Verification items for the finished model (mm, model axes). A direction names the side the tool comes from. Give positions to 0.01 mm unless a question says otherwise; leave off trailing zeros.
from build123d import *

# Parameters (mm, degrees)
SWEEP_1_PROFILE_R   = 10
SWEEP_1_PROFILE_R_2 = 7.5


with BuildPart() as part:
    # 扫描-薄件1: sweep along a curve in space
    with BuildLine() as sweep_1_path:
        Line((0, 0, 0), (0, 13.370069625, 0))
        ThreePointArc((0, 13.370069625, 0), (-3.799479767, 27.216391611, -1.753606046), (-13.925963802, 36.427367909, -6.427367909))
        Line((-51.074036198, 53.572632091, -23.572632091), (-13.925963802, 36.427367909, -6.427367909))
        ThreePointArc((-65, 60, -46.629930375), (-61.200520233, 58.246393954, -32.783608389), (-51.074036198, 53.572632091, -23.572632091))
        Line((-65, 60, -46.629930375), (-65, 60, -50))
    # 扫描-薄件1 profile (on start of the path) → 扫描-薄件1 (sweep)
    with BuildSketch(Plane(origin=(0, 0, 0), x_dir=(1, 0, 0), z_dir=(0, 1, 0))):
        Circle(SWEEP_1_PROFILE_R)
        Circle(SWEEP_1_PROFILE_R_2, mode=Mode.SUBTRACT)
    sweep(path=sweep_1_path.line)


solid = part.part
(1) Set-up check for faces 4 (the cylindrical face through (-7.493, 6.779, -0.33)), 5 (the flat face through (7, 0, 4)): record each of +Z, -Z, +X, -X, +Y, -Y from which the full face is reachable in a straight line by a thin tool's end or side.
Solved:
face 4: -Y
face 5: +Z, -Z, +X, -X, -Y
(2) Scan lines: line 1 (Z direction, x = 0, y = 7.25); line 2 (X direction, y = 60, z = -48). Record each from-to range of solid material in increasing order.
Solved:
line 1: z = -10 to -7.5, 7.5 to 10
line 2: x = -75 to -72.5, -57.5 to -55
(3) Go/stop test with flat-tipped pins: pin 1 (4 mm diameter, centred on y = 59.5, z = -26.5, fed in from +X); pin 2 (4 mm diameter, centred on x = -49, y = 44.5, fed in from +Z); pin 3 (19.5 mm diameter, centred on x = 0, z = 0, fed in from +Y); pin 4 (17.5 mm diameter, centred on x = -65, y = 60, fed in from -Z). Record where each tip stops, or that it passes through.
Solved:
pin 1: stops at x = -39.64
pin 2: stops at z = -11.81
pin 3: stops at y = 44.87
pin 4: stops at z = -50
(4) Release check for a two-part mould opening along X. For faces 1 (the flat face through (-69, 67, -50)), 2 (the cylindrical face through (-58.169, 52.696, -48.339)), 3 (the cylindrical face through (-69.5, 54, -48.3)) record: pulls with the +X half, pulls with the -X half, needs draft (parallel to the pull), parting line crosses it, or undercut.
Solved:
face 1: needs draft
face 2: parting line crosses it
face 3: undercut
